Could you check a few things on this model? Use its own coordinates, in mm. A direction names the side the tool comes from. Give positions to 0.01 mm unless a question says otherwise; leave off trailing zeros. Loops run counter-clockwise (first coordinate to the right, second up) from the corner with the lowest first, then second, coordinate; pieces in that order, holes last. Notation, with made-up numbers: (-25, 62) -> (-21, 62) arc R17 ccw to (-21, 69) -> close; hole circle Ø11 at (88, 12.25). An arc over 180 degrees is marked (long way). Write each question's results on one line, items separated by ' | '. Start each with the question number.
Q1. If we section it at C-C, the plane x = 1362: List the corners of the cut face in (y, z) for me.
Q2. Which directions (+Z, -Z, +X, -X, +Y, -Y) give clear straight access to the entire face, cutting with the end or side of a thin tool? Please do faces 1 (the face through (909.074, 384.373, 1468.722)), 2 (the face through (1724.15, 75.56, 78.52)).
Q3. If I drill on line 1 along X through (y, z) = (17.5, 98.5), over which ranges is the centre line in solid material (lowest first)?
Q4. Will these pins go through, and if not, where does the flat tip stop? P1, Ø2, axis at y = 70.5, z = 724.5, coming from the -X side; P2, Ø6, axis at y = 21, z = 160, coming from the +X side.
Q5. If we section it at A-A, the plane z = 503: List the corners of the cut face in (x, y) for me (1 decimal).
Q6. We'd pull the mould along Z, two halves only. Please class faces 3 (the face through (1796.51, 3.28, 30.07)), 4 (the face through (909, 395, 1500)), 5 (the face through (82.744, 75.023, 1419.929)), 6 (the face through (909, 389, 1450)): released by +Z, released by -Z, zero draft, split by the parting line, or undercut.
Q7. If we section it at B-B, the plane y = 228: List the corners of the cut face in (x, z) for me, plus the area to 3 significant figures.
from build123d import *

# Parameters (mm, degrees)
BOSS_EXTRUDE4_DEPTH = 1500
FILLET2_R           = 100
CUT_EXTRUDE1_DEPTH  = 1400
FILLET3_R           = 100


with BuildPart() as part:
    # Sketch1 → Boss-Extrude4 (new body)
    with BuildSketch(Plane.XY):
        with BuildLine():
            Line((1835.310496497, -2.480275435), (1799.765613012, -30.447060895))
            ThreePointArc((1799.765613012, -30.447060895), (904.320634181, 384.38013336), (9.35701304, -31.484541797))
            Line((9.35701304, -31.484541797), (-24.735019353, -1.799246648))
            ThreePointArc((-24.735019353, -1.799246648), (905.445806615, 429.580248582), (1835.310496497, -2.480275435))
        make_face()
    extrude(amount=BOSS_EXTRUDE4_DEPTH)

    # Fillet2
    fillet2_edges = [part.edges().sort_by_distance(p)[0] for p in [
        (1817.538054755, -16.463668165, 1500),
        (-7.689003156, -16.641894223, 1500),
        (1817.538054755, -16.463668165, 0),
        (-7.689003156, -16.641894223, 0),
    ]]
    fillet(fillet2_edges, radius=FILLET2_R)

    # Sketch2 → Cut-Extrude1 (cut)
    with BuildSketch(Plane.XY.offset(50)):
        with BuildLine():
            Line((1767.508699471, 71.415320952), (1731.731952363, 43.266104728))
            ThreePointArc((1731.731952363, 43.266104728), (904.184365492, 384.380046478), (77.112203072, 42.114991378))
            Line((77.112203072, 42.114991378), (42.942511203, 71.867907736))
            ThreePointArc((42.942511203, 71.867907736), (905.319541026, 429.580288265), (1767.508699471, 71.415320952))
        make_face()
    extrude(amount=CUT_EXTRUDE1_DEPTH, mode=Mode.SUBTRACT)

    # Fillet3
    fillet3_edges = [part.edges().sort_by_distance(p)[0] for p in [
        (60.027357138, 56.991449557, 50),
        (1749.620325917, 57.34071284, 50),
        (60.027357138, 56.991449557, 1450),
        (1749.620325917, 57.34071284, 1450),
    ]]
    fillet(fillet3_edges, radius=FILLET3_R)


solid = part.part
Final values:
1) outline: (291.64, 0) -> (340.56, 0) -> (340.56, 50) -> (291.64, 50) -> close; (291.64, 1450) -> (340.56, 1450) -> (340.56, 1500) -> (291.64, 1500) -> close
2) face 1: +Z, -Z, -Y | face 2: +Y
3) line 1: x = -8.07 to 53.14, 1756.86 to 1818.07
4) P1: stops at x = 40.59 | P2: stops at x = 1817.62
5) outline: (-24.7, -1.8) -> (9.4, -31.5) arc R1172.4 cw to (77.1, 42.1) -> (42.9, 71.9) arc R1217.6 ccw to start; (1731.7, 43.3) arc R1172.4 cw to (1799.8, -30.4) -> (1835.3, -2.5) arc R1217.6 ccw to (1767.5, 71.4) -> close
6) face 3: released by -Z | face 4: released by +Z | face 5: undercut | face 6: undercut
7) outline: (233.99, 0) -> (320, 0) -> (320, 50) -> (233.99, 50) -> close; (233.99, 1450) -> (320, 1450) -> (320, 1500) -> (233.99, 1500) -> close; (1490, 0) -> (1576.01, 0) -> (1576.01, 50) -> (1490, 50) -> close; (1490, 1450) -> (1576.01, 1450) -> (1576.01, 1500) -> (1490, 1500) -> close | area: 17,200 mm²
